Part model, mm, in its own coordinate system. Give positions to 0.01 mm unless a question says otherwise; leave off trailing zeros. Write each loop counter-clockwise with the first axis right and the second up, starting at its lowest first coordinate (ties: lowest second). Pieces come first, ordered by that corner, then holes. Notation, with made-up numbers: M -8.5,-17 L 10.5,-17 A27 cw 10.5,2 Z; hole C 85.25,26.25 d2. An arc over 180 degrees is marked long. Use CSV: the item, a comma, the result in double quotes. Start each with the question number.
1. Drop flat-ended pins along their axis: pin 1 Ø1.5 at (x, y) = (-154.5, 1.5) entering from -Z; pin 2 Ø5 at (x, z) = (0, 292.1) entering from +Y; pin 3 Ø6 at (x, z) = (292.1, 0) entering from +Y. Give the stop position or say it passes through.
2. Band-saw the part on C-C, the plane x = 256. List the corners of the cut face in (y, z) (3 decimals), then the cut area to 3 significant figures.
3. Band-saw the part on A-A, the plane y = 2.45. Count the separate pieces of the cut face and the enclosed holes in it, then the cut area to 3 significant figures.
4. Drill centre lines: line 1 along X through (y, z) = (1.7, -219); line 2 along X through (y, z) = (1.2, -5); line 3 along X through (y, z) = (1.25, 110.5). Where is each one in solid material? Low to high. Write a range as from..to.
5. Band-saw the part on B-B, the plane z = 133. List the corners of the cut face in (x, y) (3 decimals), then the cut area to 3 significant figures.
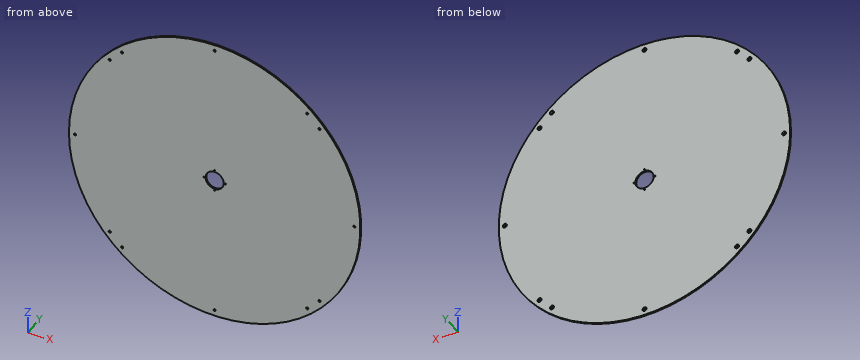
Autodesk Inventor part; units mm, degrees
ref_plane "YZ Plane" through (0, 0, 0) normal (1, 0, 0) x (0, 1, 0)
ref_plane "XZ Plane" through (0, 0, 0) normal (0, 1, 0) x (-1, 0, 0)
ref_plane "XY Plane" through (0, 0, 0) normal (0, 0, 1) x (1, 0, 0)
sketch "Sketch1" plane through (0, 0, 0) normal (0, 1, 0) x (-1, 0, 0)
  circle A0 centre (0, 0) radius 304.8
  dimension "d0" = 609.6
extrude "Extrusion1" add sketch "Sketch1" along normal blind 3.175
sketch "Sketch2" plane through (0, 3.175, 0) normal (0, 1, 0) x (1, 0, 0)
  circle A0 centre (0, 0) radius 304.8
  circle A1 centre (0, 0) radius 19.05
  dimension "d3" = 38.1
extrude "Extrusion2" cut sketch "Sketch2" against normal blind 3.175 contours A1
sketch "Sketch3" plane through (0, 3.175, 0) normal (0, 1, 0) x (1, 0, 0)
  circle A0 centre (0, 0) radius 19.05
  circle A1 centre (0, 292.1) radius 4.6302
  dimension "d6" = 292.1
hole "Hole1" at (0, 3.175, -292.1) direction (0, -1, 0) diameter 4.4958 end through all countersink diameter 8.4328 countersink angle 82
pattern_circular "Circular Pattern1" count 4 over 360 about axis through (0, 3.175, 0) along (0, -1, 0) of "Hole1"
sketch "Sketch4" plane through (0, 3.175, 0) normal (0, 1, 0) x (1, 0, 0)
  circle A0 centre (0, 0) radius 304.8
  line L0 (0, 0) -> (304.8, 0) construction
  line L1 (0, 0) -> (206.5459, 206.5459) construction
  line L2 (193.6323, 219.4595) -> (-44.0898, -18.2626) construction
  line L3 (-44.0898, -18.2626) -> (304.8, -18.2626) construction
  line L4 (219.4595, 193.6323) -> (44.0898, 18.2626) construction
  line L5 (44.0898, 18.2626) -> (304.8, 18.2626) construction
  circle A1 centre (193.6323, 219.4595) radius 4.0648
  circle A2 centre (219.4595, 193.6323) radius 4.0772
  dimension "d20" = 292.1
  dimension "d21" = 45
  dimension "d22" = 18.2626
  dimension "d23" = 18.2626
hole "Hole2" at (193.6323, 3.175, -219.4595) at (219.4595, 3.175, -193.6323) direction (0, -1, 0) diameter 4.4958 end through all countersink diameter 8.4328 countersink angle 82
pattern_circular "Circular Pattern2" count 4 over 360 about axis through (0, 3.175, 0) along (0, -1, 0) of "Hole2"
sketch "Sketch5" plane through (0, 3.175, 0) normal (0, 1, 0) x (1, 0, 0)
  circle A0 centre (0, 0) radius 19.05
  circle A1 centre (0, 22.225) radius 4.7781
  dimension "d34" = 22.225
hole "Hole3" at (0, 3.175, -22.225) direction (0, -1, 0) diameter 2.438 depth 8 tip angle 118
pattern_circular "Circular Pattern3" count 4 over 360 about axis through (0, 3.175, 0) along (0, -1, 0) of "Hole3"
properties part number "2f1bd" material "Aluminum 6061"
Output:
1,pin 1,"stops at z = -263.18"
1,pin 2,"stops at y = 1.2"
1,pin 3,"stops at y = 1.78"
2,outline,"M 0,-165.43 L 3.175,-165.43 L 3.175,165.43 L 0,165.43 Z"
2,area,"1,050 mm²"
3,separate pieces,"1"
3,enclosed holes,"17"
3,area,"290,000 mm²"
4,line 1,"x = -212..-196.53, -190.73..190.73, 196.53..212"
4,line 2,"x = -304.76..-18.38, 18.38..304.76"
4,line 3,"x = -284.06..284.06"
5,outline,"M -274.252,0 L 274.252,0 L 274.252,3.175 L -274.252,3.175 Z"
5,area,"1,740 mm²"
